from build123d import *

# Parameters (mm, degrees)
F1_DEPTH = 48
F0_W     = 92
F0_H     = 18
F2_DEPTH = 10
F4_DEPTH = 63
F6_DEPTH = 5
F7_DEPTH = 3
F8_R     = 6
F9_DEPTH = 55.6
F10_R    = 6


with BuildPart() as f1:
    # F0 (on Top) → F1 (new body)
    with BuildSketch(Plane.XY):
        Polygon((-31, 29.8156050886), (-46, 29.8156050886), (-46, -0.1843949114), (46, -0.1843949114), (46, 29.8156050886), (31, 29.8156050886), (21, 29.8156050886), (21, 9.8156050886), (-21, 9.8156050886), (-21, 29.8156050886), align=None)
    extrude(amount=F1_DEPTH)

    # F0 (on Top) → F2 (join)
    with BuildSketch(Plane.XY):
        with Locations((0, -9.1843949114)):
            Rectangle(F0_W, F0_H)
    extrude(amount=F2_DEPTH)

    # F3 (on face) → F4 (cut)
    with BuildSketch(Plane.XZ.offset(0.1843949114)):
        with BuildLine():
            Line((-31, 32.9128784748), (-31, 48))
            Line((-31, 48), (-36.0656386086, 48))
            ThreePointArc((-36.0656386086, 48), (-32.3002211531, 40.8702953048), (-31, 32.9128784748))
        make_face()
        with BuildLine():
            ThreePointArc((-46, 10), (-35.0834993366, 19.2198145372), (-31, 32.9128784748))
            ThreePointArc((-31, 32.9128784748), (-32.3002211531, 40.8702953048), (-36.0656386086, 48))
            Line((-36.0656386086, 48), (-46, 48))
            Line((-46, 48), (-46, 10))
        make_face()
        with BuildLine():
            Line((36.0656386086, 48), (31, 48))
            Line((31, 48), (31, 32.9128784748))
            ThreePointArc((31, 32.9128784748), (32.3002211531, 40.8702953048), (36.0656386086, 48))
        make_face()
        with BuildLine():
            ThreePointArc((36.0656386086, 48), (32.3002211531, 40.8702953048), (31, 32.9128784748))
            ThreePointArc((31, 32.9128784748), (35.0834993366, 19.2198145372), (46, 10))
            Line((46, 10), (46, 48))
            Line((46, 48), (36.0656386086, 48))
        make_face()
        with BuildLine():
            ThreePointArc((81, 32.9128784748), (63.9574168301, 56.6126573217), (36.0656386086, 48))
            Line((36.0656386086, 48), (46, 48))
            Line((46, 48), (46, 10))
            ThreePointArc((46, 10), (69.6930639376, 11.9963778114), (81, 32.9128784748))
        make_face()
    extrude(amount=-F4_DEPTH, mode=Mode.SUBTRACT)

    # F5 (on face) → F6 (join)
    with BuildSketch(Plane.XZ.offset(0.1843949114)):
        Polygon((14, 15), (0, 15), (-14, 15), (-14, 10), (14, 10), align=None)
    extrude(amount=F6_DEPTH)

    # F5 (on face) → F7 (join)
    with BuildSketch(Plane.XZ.offset(0.1843949114)):
        with BuildLine():
            Line((0, 29), (14, 29))
            ThreePointArc((14, 29), (0, 43), (-14, 29))
            Line((-14, 29), (0, 29))
        make_face()
        with BuildLine():
            ThreePointArc((0, 15), (9.8994949366, 19.1005050634), (14, 29))
            Line((14, 29), (0, 29))
            Line((0, 29), (-14, 29))
            ThreePointArc((-14, 29), (-9.8994949366, 19.1005050634), (0, 15))
        make_face()
        with BuildLine():
            Line((14, 15), (14, 29))
            ThreePointArc((14, 29), (9.8994949366, 19.1005050634), (0, 15))
            Line((0, 15), (14, 15))
        make_face()
        with BuildLine():
            ThreePointArc((0, 15), (-9.8994949366, 19.1005050634), (-14, 29))
            Line((-14, 29), (-14, 15))
            Line((-14, 15), (0, 15))
        make_face()
    extrude(amount=F7_DEPTH)

    # F8 (on face) → F9 (cut)
    with BuildSketch(Plane.XZ.offset(3.1843949114)):
        with Locations((0, 29)):
            Circle(F8_R)
    extrude(amount=-F9_DEPTH, mode=Mode.SUBTRACT)

    # F10
    f10_edges = [f1.edges().sort_by_distance(p)[0] for p in [
        (-46, -18.184395, 5),
        (46, -18.184395, 5),
    ]]
    fillet(f10_edges, radius=F10_R)


solid = f1.part
Work out the finished part from the listing and answer in its coordinate system (mm). A direction names the side the tool comes from. Coordinates: 2 decimals unless noted, no trailing zeros. Write each loop counter-clockwise with the first axis right and the second up, starting at its lowest first coordinate (ties: lowest second). Pieces come first, ordered by that corner, then holes.
1. Consider line 1 along Z through (x, y) = (0, 0.75); line 2 along X through (y, z) = (26.5, 36.5); line 3 along Z through (x, y) = (39, -13). Determine where each line is inside the solid, lowest interval first.
Results list:
line 1: z = 0 to 23, 35 to 48
line 2: x = -31 to -21, 21 to 31
line 3: z = 0 to 10
2. The part is cut by section D-D, the plane y = -1.5. Write down the section's boundary in (x, z), and give its area (3 significant figures).
Results list:
outline: (-46, 0) - (46, 0) - (46, 10) - (14, 10) - (14, 29) arc R14 ccw to (-14, 29) - (-14, 10) - (-46, 10) - close; hole circle Ø12 at (0, 29)
area: 1,650 mm2
3. The part is cut by section A-A, the plane x = 0. Write down the section's boundary in (y, z).
Results list:
outline: (-18.18, 0) - (9.82, 0) - (9.82, 23) - (-3.18, 23) - (-3.18, 15) - (-5.18, 15) - (-5.18, 10) - (-18.18, 10) - close; (-3.18, 35) - (9.82, 35) - (9.82, 48) - (-0.18, 48) - (-0.18, 43) - (-3.18, 43) - close
4. For a pull along Z with two mould halves and no side action, classify faces 1 (the flat face through (-1, -18.184, 5)), 2 (the flat face through (0, 8, 48)), 3 (the cylindrical face through (-1.301, 3.225, 23.143)) as +Z half, -Z half, draft (parallel to the pull), parting line (faces both ways), or undercut.
Results list:
face 1: draft
face 2: +Z half
face 3: undercut
5. The part is cut by section C-C, the plane z = 25. Write down the section's boundary in (x, y), and give its area (3 significant figures).
Results list:
outline: (-32.29, -0.18) - (-14, -0.18) - (-14, -3.18) - (-4.47, -3.18) - (-4.47, 9.82) - (-21, 9.82) - (-21, 29.82) - (-32.29, 29.82) - close; (4.47, -3.18) - (14, -3.18) - (14, -0.18) - (32.29, -0.18) - (32.29, 29.82) - (21, 29.82) - (21, 9.82) - (4.47, 9.82) - close
area: 1,060 mm2
6. The part is cut by section B-B, the plane y = 21.5. Write down the section's boundary in (x, z).
Results list:
outline: (-46, 0) - (-21, 0) - (-21, 48) - (-31, 48) - (-31, 32.91) arc R25 cw to (-46, 10) - close; (21, 0) - (46, 0) - (46, 10) arc R25 cw to (31, 32.91) - (31, 48) - (21, 48) - close
7. Flat-ended cylindrical pins translate along their axes: pin 1 (19 mm diameter, centred on x = 0, z = 29, fed in from -Y); pin 2 (2.5 mm diameter, centred on y = -2, z = 15, fed in from +X); pin 3 (1 mm diameter, centred on y = 23, z = 21, fed in from -X); pin 4 (1 mm diameter, centred on x = 11, y = 2, fed in from -Z). Find the tip coordinate at first contact, or state that the pin passes through.
Results list:
pin 1: stops at y = -3.18
pin 2: stops at x = 14
pin 3: stops at x = -34.3
pin 4: stops at z = 0
8. For faces 4 (the cylindrical face through (0, -2, 43)), 5 (the flat face through (31, 15, 41)), 6 (the flat face through (-14, -2, 18)), 7 (the flat face through (-31, 15, 40)), determine the directions among +Z, -Z, +X, -X, +Y, -Y from which every point of the face is accessible in a straight line to the end or side of a thin tool.
Results list:
face 4: +Z, -Y
face 5: +Z, +X, +Y, -Y
face 6: +Z, -X, -Y
face 7: +Z, -X, +Y, -Y
